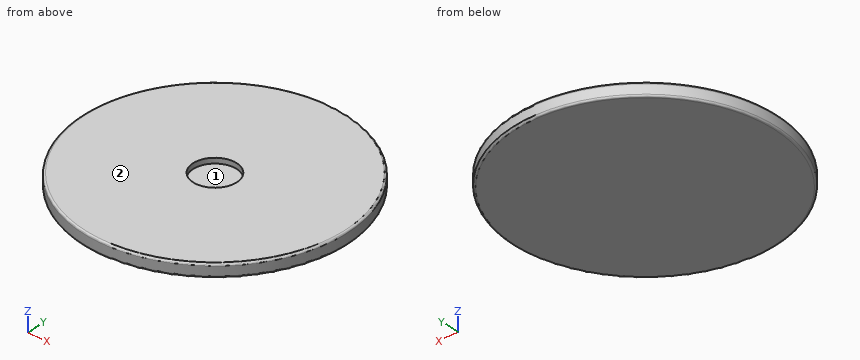
from build123d import *

# Parameters (mm, degrees)
F0_R     = 10
F1_DEPTH = 1
F2_R     = 0.15
F3_R     = 1.65
F4_DEPTH = 0.4


# Not quite as in the source:
# - a feature names something its author has since deleted; it is built from what else it names


with BuildPart() as f1:
    # F0 (on Top) → F1 (new body)
    with BuildSketch(Plane.XY):
        Circle(F0_R)
    extrude(amount=F1_DEPTH)

    # F2
    f2_edges = [f1.edges().sort_by_distance(p)[0] for p in [
        (-10, 0, 1),
        (-10, 0, 0),
    ]]
    fillet(f2_edges, radius=F2_R)

    # F3 (on face) → F4 (cut)
    with BuildSketch(Plane.XY.offset(1)):
        Circle(F3_R)
    extrude(amount=-F4_DEPTH, mode=Mode.SUBTRACT)


solid = f1.part
Source: CAD feature listing. Evaluate the final solid. Frame: model axes, mm. Face numbers are marked on the shaded views. Coordinates: 2 decimals unless noted, no trailing zeros. Loops run counter-clockwise (first coordinate to the right, second up) from the corner with the lowest first, then second, coordinate; pieces in that order, holes last. Notation, with made-up numbers: M -7.75,85 L 39.25,85 A12 cw 39.25,99 Z; hole C 68.5,55 d8. An arc over 180 degrees is marked long. Answer in a Markdown table with one row per item.
Q1. Draft query along Y for the marked faces 1 and 2. Return one class per face: pulls with the +Y half, pulls with the -Y half, needs draft (parallel to the pull), parting line crosses it, or undercut.
Answers below:
| item | result |
|---|---|
| face 1 | undercut |
| face 2 | needs draft |
Q2. First-contact query: pin 1 (2 mm diameter, centred on x = 0, y = 0, fed in from +Z). Flat tip, straight axial feed; report the tip coordinate or a pass-through.
Answers below:
| item | result |
|---|---|
| pin 1 | stops at z = 0.6 |
Q3. Section A-A on x = 0. Return the cut outline in (y, z), plus the area to 3 significant figures.
Answers below:
| item | result |
|---|---|
| outline | M -10,0.15 A0.15 ccw -9.85,0 L 9.85,0 A0.15 ccw 10,0.15 L 10,0.85 A0.15 ccw 9.85,1 L 1.65,1 L 1.65,0.6 L -1.65,0.6 L -1.65,1 L -9.85,1 A0.15 ccw -10,0.85 Z |
| area | 18.7 mm^2 |
Q4. Section C-C on z = 0.3. Return the cut outline in (x, y), plus the area to 3 significant figures.
Answers below:
| item | result |
|---|---|
| outline | C 0,0 d20 |
| area | 314 mm^2 |
Q5. Ray query, probe 1 along Y at (x, z) = (0, 0.7); probe 2 along Y at (x, z) = (-0.25, 0.25); probe 3 along Y at (x, z) = (-1.25, 0.8). Return the intervals inside material, ascending. Write a range as from..to.
Answers below:
| item | result |
|---|---|
| probe 1 | y = -10..-1.65, 1.65..10 |
| probe 2 | y = -10..10 |
| probe 3 | y = -9.92..-1.08, 1.08..9.92 |
